```python
from build123d import *

# Parameters (mm, degrees)
BOSS_EXTRUDE1_DEPTH = 8
SKETCH3_R           = 2.5
BOSS_EXTRUDE2_DEPTH = 5


with BuildPart() as part:
    # Sketch1 → Boss-Extrude1 (new body)
    with BuildSketch(Plane.XY):
        Polygon((1.732050808, 3), (-1.732050808, 3), (-3.464101615, 0), (-1.732050808, -3), (1.732050808, -3), (3.464101615, 0), align=None)
    extrude(amount=BOSS_EXTRUDE1_DEPTH)

    # Sketch2 → Cut-Revolve1 (revolve, cut)
    with BuildSketch(Plane(origin=(0, 0, 0), x_dir=(1, 0, 0), z_dir=(0, 1, 0))):
        Polygon((-0.508, 0), (-3.464101615, -3.52294472), (-3.464101615, 0), align=None)
    revolve(axis=Axis((0, 0, 0), (0, 0, 1)), mode=Mode.SUBTRACT)

    # Sketch3 → Boss-Extrude2 (add)
    with BuildSketch(Plane.XY.offset(8)):
        Circle(SKETCH3_R)
    extrude(amount=BOSS_EXTRUDE2_DEPTH)

    # Sketch4 → Cut-Revolve2 (revolve, cut)
    with BuildSketch(Plane(origin=(0, 0, 0), x_dir=(1, 0, 0), z_dir=(0, 1, 0))):
        Polygon((0, 0), (0, -13), (-1, -13), (-1, -1.638256659), (-0.2, -1.212889113), (-0.2, 0), align=None)
    revolve(axis=Axis((0, 0, 0), (0, 0, 1)), mode=Mode.SUBTRACT)


solid = part.part
```
Model file for the job. Use its own axes, mm. A direction names the side the tool comes from. Coordinates: 2 decimals unless noted, no trailing zeros. Order: outer loops, then holes, each group sorted by start corner. A loop starts at its lowest first (then second) coordinate and runs counter-clockwise, first axis right, second up. Notation, with made-up numbers: (-3, 57.25) - (50, 57.25) arc R23 ccw to (50, 76.25) - close; hole circle Ø11 at (83, -37). An arc over 180 degrees is marked (long way). Return JSON: item names as keys, results as strings. Group by question number.
1) Saw through at D-D, the plane z = 2.25. Write the cut outline in (x, y).
2) Saw through at B-B, the plane z = 6.25. Write the cut outline in (x, y).
3) Saw through at C-C, the plane z = 11. Write the cut outline in (x, y).
4) Saw through at A-A, the plane x = 0. Write the cut outline in (y, z), plus the area to 3 significant figures.
5) Mould opens along X. For faces 1 (the conical face through (0.221, 0.997, 0.612)), 2 (the flat face through (-2.6, 1.5, 5.4)), 3 (the cylindrical face through (0, 1, 7)), 4 (the flat face through (0, 3, 5)) say: released by +X, released by -X, zero draft, split by the parting line, or undercut.
6) Probe line 1 (Y direction, x = -0.5, z = 4.25); line 2 (Y direction, x = -0.5, z = 1.75); line 3 (X direction, y = 0, z = 0.7). List the from-to ranges inside material, lowest first. Write a range as from..to.
7) Tool access for faces 5 (the flat face through (-2.6, -1.5, 5.4)), 6 (the cylindrical face through (-0.54, -2.44, 10.46)): list every direction of +Z, -Z, +X, -X, +Y, -Y with a clear straight run to the whole face (end or side of a thin tool).
8) Flat gauge pins, fed straight in: P1, Ø2, axis at y = -2.5, z = 8, coming from the +X side; P2, Ø1.5, axis at x = -2.5, y = -1, coming from the -Z side. Where does each tip first touch, or does it go through?
Values found:
{
 "1": {"outline": "circle Ø4.79 at (0, 0); hole circle Ø2 at (0, 0)"},
 "2": {"outline": "(-3.46, 0) - (-1.73, -3) - (1.73, -3) - (3.46, 0) - (1.73, 3) - (-1.73, 3) - close; hole circle Ø2 at (0, 0)"},
 "3": {"outline": "circle Ø5 at (0, 0); hole circle Ø2 at (0, 0)"},
 "4": {"outline": "(-3, 2.97) - (-0.51, 0) - (-0.2, 0) - (-0.2, 1.21) - (-1, 1.64) - (-1, 13) - (-2.5, 13) - (-2.5, 8) - (-3, 8) - close; (0.2, 0) - (0.51, 0) - (3, 2.97) - (3, 8) - (2.5, 8) - (2.5, 13) - (1, 13) - (1, 1.64) - (0.2, 1.21) - close", "area": "41.9 mm²"},
 "5": {"face 1": "split by the parting line", "face 2": "released by -X", "face 3": "undercut", "face 4": "zero draft"},
 "6": {"line 1": "y = -3..-0.87, 0.87..3", "line 2": "y = -1.91..-0.87, 0.87..1.91", "line 3": "x = -1.1..-0.2, 0.2..1.1"},
 "7": {"face 5": "+Z, -Z, -X, -Y", "face 6": "+Z"},
 "8": {"P1": "stops at x = 2.6", "P2": "stops at z = 1.71"}
}
